Can you work these out from the model? Positions are in its coordinate system, mm. Face numbers are marked on the shaded views. A direction names the side the tool comes from. Round coordinates to 2 decimals unless told otherwise and drop trailing zeros. Loops run counter-clockwise (first coordinate to the right, second up) from the corner with the lowest first, then second, coordinate; pieces in that order, holes last.
(1) Will these pins go through, and if not, where does the flat tip stop? pin 1 Ø2.5 at (y, z) = (32, 2.5) entering from +X; pin 2 Ø4.5 at (x, y) = (6.5, 0) entering from -Z; pin 3 Ø1.9 at (y, z) = (-22.5, 22.5) entering from -X; pin 4 Ø8 at (x, y) = (6.5, 20.5) entering from +Z.
(2) I want a section at A-A on z = 22.5. Write out the boundary of the cut face in (x, y).
(3) Which directions (+Z, -Z, +X, -X, +Y, -Y) give clear straight access to the entire face, cutting with the end or side of a thin tool? Please do the marked faces 1 and 2.
(4) I want a section at B-B on y = 22.5. Write out the boundary of the cut face in (x, z), plus the area to 3 significant figures.
(5) If I drill on line 1 along Y through (x, z) = (-6.5, 22.5); line 2 along X through (y, z) = (-17, 26); line 3 along Z through (x, y) = (2, 22.5), over which ranges is the centre line in solid material (lowest first)?
(6) I want a section at C-C on z = 9. Write out the boundary of the cut face in (x, y).
(7) I want a section at D-D on x = 3.75. Write out the boundary of the cut face in (y, z).
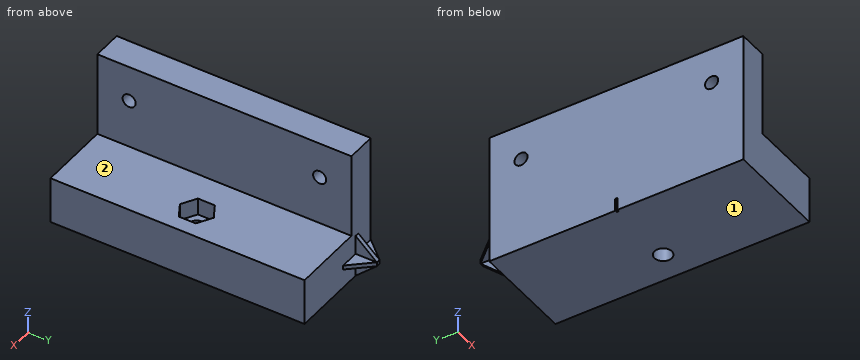
Autodesk Inventor part; units mm, degrees
ref_plane "YZ Plane" through (0, 0, 0) normal (1, 0, 0) x (0, 1, 0)
ref_plane "XZ Plane" through (0, 0, 0) normal (0, 1, 0) x (-1, 0, 0)
ref_plane "XY Plane" through (0, 0, 0) normal (0, 0, 1) x (1, 0, 0)
sketch "Skizze1" plane through (0, 0, 0) normal (0, 0, 1) x (1, 0, 0)
  line L0 (-13.5, 30) -> (13.5, 30)
  line L1 (13.5, 30) -> (13.5, -30)
  line L2 (13.5, -30) -> (-13.5, -30)
  line L3 (-13.5, -30) -> (-13.5, 30)
  line L4 (-13.5, 30) -> (13.5, -30) construction
  line L5 (13.5, 30) -> (-13.5, -30) construction
  point P0 (0, 0)
  dimension "d0" = 27
  dimension "d1" = 60
extrude "Extrusion1" add sketch "Skizze1" along normal blind 11
sketch "Skizze2" plane through (0, 0, 11) normal (0, 0, 1) x (1, 0, 0)
  line L0 (13.5, 30) -> (-13.5, 30)
  line L1 (-13.5, -30) -> (13.5, -30)
  line L2 (-13.5, 30) -> (-3.5, 30)
  line L3 (-3.5, 30) -> (-3.5, -30)
  line L4 (-3.5, -30) -> (-13.5, -30)
  line L5 (-13.5, -30) -> (-13.5, 30)
  point P0 (0, 0)
  dimension "d4" = 10
extrude "Extrusion2" add sketch "Skizze2" along normal blind 20
sketch "Skizze3" plane through (-3.5, -30, 11) normal (1, 0, 0) x (0, 0, -1)
  line L0 (0, 60) -> (0, 0) construction
  line L1 (0, 60) -> (-20, 60) construction
  line L2 (-20, 0) -> (-20, 60) construction
  line L3 (0, 0) -> (-20, 0) construction
  line L4 (0, 60) -> (0, 0)
  line L5 (0, 30) -> (-11.5, 30) construction
  line L6 (-11.5, 30) -> (-11.5, 52.5) construction
  line L7 (-11.5, 30) -> (-11.5, 7.5) construction
  circle A0 centre (-11.5, 7.5) radius 1.55
  circle A1 centre (-11.5, 52.5) radius 1.55
  point P0 (11, 30)
  dimension "d7" = 11.5
  dimension "d8" = 22.5
  dimension "d9" = 22.5
  dimension "d10" = 3.1
  dimension "d11" = 3.1
extrude "Extrusion3" cut sketch "Skizze3" against normal through all
sketch "Skizze4" plane through (-13.5, -30, 0) normal (-1, 0, 0) x (0, 0, 1)
  circle A0 centre (22.5, 7.5) radius 1.55
  circle A1 centre (22.5, 52.5) radius 1.55
  line L0 (0, 0) -> (0, 60)
  line L1 (0, 0) -> (31, 0)
  line L2 (31, 60) -> (31, 0)
  line L3 (0, 60) -> (31, 60)
  point P0 (0, 30)
extrude "Extrusion4" cut sketch "Skizze4" against normal blind 3
sketch "Skizze5" plane through (-10.5, -30, 0) normal (-1, 0, 0) x (0, 0, 1)
  line L0 (-3, 30.25) -> (3, 30.25)
  line L1 (3, 30.25) -> (3, 29.75)
  line L2 (3, 29.75) -> (-3, 29.75)
  line L3 (-3, 29.75) -> (-3, 30.25)
  line L4 (-3, 30.25) -> (3, 29.75) construction
  line L5 (3, 30.25) -> (-3, 29.75) construction
  point P0 (0, 30)
  dimension "d16" = 6
  dimension "d17" = 0.5
extrude "Extrusion5" cut sketch "Skizze5" against normal blind 0.5
sketch "Skizze6" plane through (0, 0, 11) normal (0, 0, 1) x (1, 0, 0)
  line L0 (-3.5, -30) -> (-3.5, 30)
  line L1 (-3.5, 0) -> (6.5, 0)
  circle A0 centre (6.5, 0) radius 2.05
  point P0 (0, 0)
  dimension "d20" = 10
  dimension "d21" = 4.1
extrude "Extrusion6" cut sketch "Skizze6" against normal through all
sketch "Skizze7" plane through (0, 0, 11) normal (0, 0, 1) x (1, 0, 0)
  circle A0 centre (6.5, 0) radius 2.05
  line L0 (6.5, 0) -> (6.5, 4)
  line L1 (6.5, 0) -> (14.5, 0) construction
  line L2 (6.5, 4) -> (9.9641, 2)
  line L3 (9.9641, 2) -> (9.9641, -2)
  line L4 (9.9641, -2) -> (6.5, -4)
  line L5 (6.5, -4) -> (3.0359, -2)
  line L6 (3.0359, -2) -> (3.0359, 2)
  line L7 (3.0359, 2) -> (6.5, 4)
  point P0 (0, 0)
  dimension "d24" = 4
extrude "Extrusion7" cut sketch "Skizze7" against normal blind 4
ref_plane "Arbeitsebene1" through (6.5, 0, 11) normal (0, 0, 1) x (1, 0, 0)
ref_plane "Arbeitsebene2" through (6.5, 0, 11) normal (0, 1, 0) x (1, 0, 0)
ref_plane "Arbeitsebene3" through (6.5, 0, 11) normal (1, 0, 0) x (0, 0, -1)
sketch "Skizze11" plane through (13.5, 30, 11) normal (0, 1, 0) x (1, 0, 0)
  line L0 (-24, 11) -> (-24, -20) construction
  line L1 (-17, -20) -> (-24, -20) construction
  line L2 (-17, 0) -> (-17, -20) construction
  line L3 (0, 0) -> (-17, 0) construction
  line L4 (0, 11) -> (0, 0) construction
  line L5 (-24, 11) -> (0, 11) construction
  line L6 (0, 11) -> (-24, 11)
  line L7 (-24, 11) -> (-14, 11) construction
  line L8 (-14, 11) -> (-14, 1) construction
  line L9 (-14, 1) -> (-24, 1) construction
  line L10 (-24, 1) -> (-24, 11) construction
  line L11 (-24, 11) -> (-24, -20)
  line L12 (-14, 6.5) -> (-24, 6.5)
  line L13 (-24, 6.5) -> (-24, 5.5)
  line L14 (-24, 5.5) -> (-14, 5.5)
  line L15 (-14, 5.5) -> (-14, 6.5)
  line L16 (-14, 6.5) -> (-24, 5.5) construction
  line L17 (-24, 6.5) -> (-14, 5.5) construction
  line L18 (-18.5, 11) -> (-19.5, 11)
  line L19 (-19.5, 11) -> (-19.5, 1)
  line L20 (-19.5, 1) -> (-18.5, 1)
  line L21 (-18.5, 1) -> (-18.5, 11)
  line L22 (-18.5, 11) -> (-19.5, 1) construction
  line L23 (-19.5, 11) -> (-18.5, 1) construction
  point P0 (-13.5, 11)
  point P1 (-19, 6)
  point P2 (-19, 6)
  dimension "d46" = 10
  dimension "d47" = 10
extrude "Extrusion11" add sketch "Skizze11" along normal blind 5 contours L21 L12 L19 L6 | L21 L14 L19 L12 | L12 L15 L14 L21 | L19 L14 L11 L12 | L21 L20 L19 L14
sketch "Skizze12" plane through (-6, 30, 5.5) normal (-1, 0, 0) x (0, 0, 1)
  line L0 (0, 5) -> (0, 0)
  line L1 (4.5, 0) -> (0, 0)
  line L2 (4.5, 0) -> (4.5, 5)
  line L3 (0, 5) -> (4.5, 5)
  line L4 (-1, 0) -> (-1, 5)
  line L5 (-5.5, 5) -> (-1, 5)
  line L6 (-5.5, 0) -> (-5.5, 5)
  line L7 (-1, 0) -> (-5.5, 0)
  line L8 (0, 0) -> (0, 5)
  line L9 (4.5, 0) -> (4.5, 5)
  line L10 (0, 5) -> (4.5, 5)
  line L11 (4.5, 5) -> (4.5, 0)
  line L12 (4.5, 0) -> (0, 5)
  line L13 (-5.5, 5) -> (-1, 5)
  line L14 (-5.5, 5) -> (-1, 5)
  line L15 (-5.5, 0) -> (5.5, 0)
  line L16 (-1, 5) -> (-5.5, 0)
  line L17 (-5.5, 0) -> (-5.5, 5)
  point P0 (-5.5, -30)
extrude "Extrusion12" cut sketch "Skizze12" against normal up to surface (1 mm away) contours L3 L2 L12 | L16 L6 L5
sketch "Skizze13" plane through (-10.5, 30, 5.5) normal (0, 0, 1) x (1, 0, 0)
  line L0 (4.5, 5) -> (4.5, 0)
  line L1 (0, 5) -> (4.5, 5)
  line L2 (0, 0) -> (0, 5)
  line L3 (4.5, 0) -> (0, 0)
  line L4 (5.5, 0) -> (5.5, 5)
  line L5 (10, 0) -> (5.5, 0)
  line L6 (10, 0) -> (10, 5)
  line L7 (5.5, 5) -> (10, 5)
  line L8 (4.5, 0) -> (4.5, 5)
  line L9 (4.5, 5) -> (0, 0)
  line L10 (0, 5) -> (4.5, 5)
  line L11 (0, 5) -> (4.5, 5)
  line L12 (0, 5) -> (0, 0)
  line L13 (5.5, 5) -> (5.5, 0)
  line L14 (5.5, 0) -> (5.5, 5)
  line L15 (10, 5) -> (5.5, 5)
  line L16 (5.5, 5) -> (10, 5)
  line L17 (5.5, 5) -> (10, 0)
  line L18 (10, 0) -> (10, 5)
  line L19 (10, 5) -> (10, 0)
  point P0 (10.5, -30)
extrude "Extrusion13" cut sketch "Skizze13" against normal up to surface (1 mm away) contours L9 L2 L1 | L7 L6 L17
properties part number "cam_holder_hog_part" material "Acetalharz, Schwarz"
Filled sheet:
1. pin 1: stops at x = -5
1. pin 2: stops at z = 0
1. pin 3: passes through
1. pin 4: stops at z = 11
2. outline: (-10.5, -30) - (-3.5, -30) - (-3.5, -24.05) - (-10.5, -24.05) - close; (-10.5, -20.95) - (-3.5, -20.95) - (-3.5, 20.95) - (-10.5, 20.95) - close; (-10.5, 24.05) - (-3.5, 24.05) - (-3.5, 30) - (-10.5, 30) - close
3. face 1: -Z, +X, -X, +Y, -Y
3. face 2: +Z, +X, +Y, -Y
4. outline: (-10.5, 0) - (13.5, 0) - (13.5, 11) - (-3.5, 11) - (-3.5, 20.95) - (-10.5, 20.95) - close; (-10.5, 24.05) - (-3.5, 24.05) - (-3.5, 31) - (-10.5, 31) - close
4. area: 382 mm2
5. line 1: y = -30 to -24.05, -20.95 to 20.95, 24.05 to 30
5. line 2: x = -10.5 to -3.5
5. line 3: z = 0 to 11
6. outline: (-10.5, -30) - (13.5, -30) - (13.5, 30) - (-5, 30) - (-5, 31.11) - (-6, 31.11) - (-6, 30) - (-10.5, 30) - close; hole (3.04, -2) - (6.5, -4) - (9.96, -2) - (9.96, 2) - (6.5, 4) - (3.04, 2) - close
7. outline: (-30, 0) - (30, 0) - (30, 11) - (2.41, 11) - (2.41, 7) - (-2.41, 7) - (-2.41, 11) - (-30, 11) - close
